from build123d import *

# Parameters (mm, degrees)
F0_W     = 50.8
F0_H     = 50.8
F0_R     = 1.778
F0_R_2   = 11.5316
F1_DEPTH = 3.175
F2_R     = 1


with BuildPart() as f1:
    # F0 (on Top) → F1 (new body)
    with BuildSketch(Plane.XY):
        with Locations((25.4, 25.4)):
            Rectangle(F0_W, F0_H)
        with Locations((9.398, 9.398)):
            Circle(F0_R, mode=Mode.SUBTRACT)
        with Locations((25.4, 25.4)):
            Circle(F0_R_2, mode=Mode.SUBTRACT)
        with Locations((41.402, 9.398)):
            Circle(F0_R, mode=Mode.SUBTRACT)
        with Locations((9.398, 41.402)):
            Circle(F0_R, mode=Mode.SUBTRACT)
        with Locations((41.402, 41.402)):
            Circle(F0_R, mode=Mode.SUBTRACT)
    extrude(amount=F1_DEPTH)

    # F2
    f2_edges = [f1.edges().sort_by_distance(p)[0] for p in [
        (50.8, 0, 1.5875),
        (50.8, 50.8, 1.5875),
        (0, 50.8, 1.5875),
        (0, 0, 1.5875),
    ]]
    fillet(f2_edges, radius=F2_R)


solid = f1.part
Build history of the part. All positions in model axes, mm. Give positions to 0.01 mm unless a question says otherwise; leave off trailing zeros. Write each loop counter-clockwise with the first axis right and the second up, starting at its lowest first coordinate (ties: lowest second). Pieces come first, ordered by that corner, then holes. Notation, with made-up numbers: (76, 37) - (89, 37) arc R36 ccw to (89, 72) - close; hole circle Ø10 at (77.25, 3.25). An arc over 180 degrees is marked (long way). Use one line per item in the form item = value. Start each with the question number.
1. Band-saw the part on C-C on z = 1.75. Write the cut outline in (x, y).
2. Probe line 1 (Y direction, x = 41, z = 1.6); line 2 (X direction, y = 42, z = 2.85); line 3 (X direction, y = 10.5, z = 0.85). List the from-to ranges inside material, lowest first. Write a range as [from, to].
3. Band-saw the part on A-A on y = 25.4. Write the cut outline in (x, z) (3 decimals), plus the area to 3 significant figures.
4. Two-plate mould, pull along Y, no slides. Class faces 1 (the face through (9.17, 11.16, 1.57)), 2 (the face through (25, 0, 2)), 3 (the face through (0, 25, 2)): released by +Y, released by -Y, zero draft, split by the parting line, or undercut.
5. Drop a flat-ended pin along its axis: pin 1 Ø4 at (x, y) = (41.402, 41.402) entering from +Z (3 decimals). Give the stop position or say it passes through.
Conclusion:
q1.outline = (0, 1) arc R1 ccw to (1, 0) - (49.8, 0) arc R1 ccw to (50.8, 1) - (50.8, 49.8) arc R1 ccw to (49.8, 50.8) - (1, 50.8) arc R1 ccw to (0, 49.8) - close; hole circle Ø3.56 at (9.4, 9.4); hole circle Ø3.56 at (9.4, 41.4); hole circle Ø23.06 at (25.4, 25.4); hole circle Ø3.56 at (41.4, 9.4); hole circle Ø3.56 at (41.4, 41.4)
q2.line_1 = [0, 7.67], [11.13, 39.67], [43.13, 50.8]
q2.line_2 = [0, 7.72], [11.07, 39.73], [43.08, 50.8]
q2.line_3 = [0, 8], [10.79, 40.01], [42.8, 50.8]
q3.outline = (0, 0) - (13.868, 0) - (13.868, 3.175) - (0, 3.175) - close; (36.932, 0) - (50.8, 0) - (50.8, 3.175) - (36.932, 3.175) - close
q3.area = 88.1 mm²
q4.face_1 = undercut
q4.face_2 = released by -Y
q4.face_3 = zero draft
q5.pin_1 = 3.175
